CAD build for the part. Positions are in the model's coordinates, mm. A direction names the side the tool comes from. Round coordinates to 2 decimals unless told otherwise and drop trailing zeros. Loops run counter-clockwise (first coordinate to the right, second up) from the corner with the lowest first, then second, coordinate; pieces in that order, holes last.
from build123d import *

# Parameters (mm, degrees)
SKETCH1_W           = 30
SKETCH1_H           = 30
BOSS_EXTRUDE1_DEPTH = 15
SKETCH2_R           = 2.45
CUT_EXTRUDE1_DEPTH  = 46
CUT_EXTRUDE2_DEPTH  = 6.5
SKETCH4_R           = 6.4
CUT_EXTRUDE3_DEPTH  = 3.3
SKETCH5_R           = 4.95
CUT_EXTRUDE4_DEPTH  = 44.543541427
SKETCH6_R           = 1.25
FILLET1_R           = 0.5
CUT_EXTRUDE5_DEPTH  = 3.2
SKETCH9_W           = 34
SKETCH9_H           = 34
CUT_EXTRUDE7_DEPTH  = 9


with BuildPart() as part:
    # Sketch1 → Boss-Extrude1 (new body)
    with BuildSketch(Plane(origin=(0, 0, 0), x_dir=(0, 0, -1), z_dir=(1, 0, 0))):
        with Locations((15, 15)):
            Rectangle(SKETCH1_W, SKETCH1_H)
    extrude(amount=BOSS_EXTRUDE1_DEPTH)

    # Sketch2 → Cut-Extrude1 (cut, through all)
    with BuildSketch(Plane.ZY):
        with Locations((-24, 24)):
            Circle(SKETCH2_R)
        with Locations((-6, 24)):
            Circle(SKETCH2_R)
        with Locations((-6, 6)):
            Circle(SKETCH2_R)
        with Locations((-24, 6)):
            Circle(SKETCH2_R)
    extrude(amount=-CUT_EXTRUDE1_DEPTH, mode=Mode.SUBTRACT)

    # Sketch3 → Cut-Extrude2 (cut)
    with BuildSketch(Plane.ZY):
        Polygon((-7.609916554, 15), (-11.304958277, 21.4), (-18.695041723, 21.4), (-22.390083446, 15), (-18.695041723, 8.6), (-11.304958277, 8.6), align=None)
    extrude(amount=-CUT_EXTRUDE2_DEPTH, mode=Mode.SUBTRACT)

    # Sketch4 → Cut-Extrude3 (cut)
    with BuildSketch(Plane.ZY.offset(-6.5)):
        with Locations((-15, 15)):
            Circle(SKETCH4_R)
    extrude(amount=-CUT_EXTRUDE3_DEPTH, mode=Mode.SUBTRACT)

    # Sketch5 → Cut-Extrude4 (cut, through all)
    with BuildSketch(Plane.ZY.offset(-9.8)):
        with Locations((-15, 15)):
            Circle(SKETCH5_R)
    extrude(amount=-CUT_EXTRUDE4_DEPTH, mode=Mode.SUBTRACT)

    # Sketch6 → Cut-Revolve1 (revolve, cut)
    with BuildSketch(Plane.XY.offset(-15), mode=Mode.PRIVATE) as cut_revolve1_sk:
        with Locations((14.4, 23.3)):
            Circle(SKETCH6_R)
    revolve(cut_revolve1_sk.sketch.rotate(Axis((9.8, 15, -15), (-1, 0, 0)), 90), axis=Axis((9.8, 15, -15), (-1, 0, 0)), mode=Mode.SUBTRACT)

    # Fillet1
    fillet1_edges = [part.edges().sort_by_distance(p)[0] for p in [
        (0, 30, -15),
        (0, 15, -30),
        (0, 0, -15),
        (0, 15, 0),
        (7.5, 30, -30),
        (7.5, 0, -30),
    ]]
    fillet(fillet1_edges, radius=FILLET1_R)

    # Sketch7 → Cut-Extrude5 (cut)
    with BuildSketch(Plane.ZY):
        Polygon((-18.630642497, 24), (-21.315321248, 28.65), (-26.684678752, 28.65), (-29.369357503, 24), (-26.684678752, 19.35), (-21.315321248, 19.35), align=None)
        Polygon((-0.630642497, 24), (-3.315321248, 28.65), (-8.684678752, 28.65), (-11.369357503, 24), (-8.684678752, 19.35), (-3.315321248, 19.35), align=None)
        Polygon((-0.630642497, 6), (-3.315321248, 10.65), (-8.684678752, 10.65), (-11.369357503, 6), (-8.684678752, 1.35), (-3.315321248, 1.35), align=None)
        Polygon((-18.630642497, 6), (-21.315321248, 10.65), (-26.684678752, 10.65), (-29.369357503, 6), (-26.684678752, 1.35), (-21.315321248, 1.35), align=None)
    extrude(amount=-CUT_EXTRUDE5_DEPTH, mode=Mode.SUBTRACT)

    # Sketch9 → Cut-Extrude7 (cut)
    with BuildSketch(Plane(origin=(15, 0, 0), x_dir=(0, 0, -1), z_dir=(1, 0, 0))):
        with Locations((15, 15)):
            Rectangle(SKETCH9_W, SKETCH9_H)
        with BuildLine():
            ThreePointArc((10.107346068, 27.582207179), (2.146268043, 27.853731957), (2.417792821, 19.892653932))
            ThreePointArc((2.417792821, 19.892653932), (1.5, 15), (2.417792821, 10.107346068))
            ThreePointArc((2.417792821, 10.107346068), (2.146268043, 2.146268043), (10.107346068, 2.417792821))
            ThreePointArc((10.107346068, 2.417792821), (15, 1.5), (19.892653932, 2.417792821))
            ThreePointArc((19.892653932, 2.417792821), (27.853731957, 2.146268043), (27.582207179, 10.107346068))
            ThreePointArc((27.582207179, 10.107346068), (28.5, 15), (27.582207179, 19.892653932))
            ThreePointArc((27.582207179, 19.892653932), (27.853731957, 27.853731957), (19.892653932, 27.582207179))
            ThreePointArc((19.892653932, 27.582207179), (15, 28.5), (10.107346068, 27.582207179))
        make_face(mode=Mode.SUBTRACT)
    extrude(amount=-CUT_EXTRUDE7_DEPTH, mode=Mode.SUBTRACT)


solid = part.part
Item 1: Cut at C-C (z = -25.5). List the corners of the cut face in (x, y).
Verdict:
outline: (0, 0.5) arc R0.5 ccw to (0.5, 0) - (6, 0) - (6, 0.76) - (15, 0.76) - (15, 4.06) - (3.2, 4.06) - (3.2, 1.35) - (0, 1.35) - close; (0, 10.65) - (3.2, 10.65) - (3.2, 7.94) - (15, 7.94) - (15, 22.06) - (3.2, 22.06) - (3.2, 19.35) - (0, 19.35) - close; (0, 28.65) - (3.2, 28.65) - (3.2, 25.94) - (15, 25.94) - (15, 29.24) - (6, 29.24) - (6, 30) - (0.5, 30) arc R0.5 ccw to (0, 29.5) - close
Item 2: Cut at A-A (x = 5). List the corners of the cut face in (y, z), plus the area to 3 significant figures.
Verdict:
outline: (0, -29.5) arc R0.5 ccw to (0.5, -30) - (29.5, -30) arc R0.5 ccw to (30, -29.5) - (30, 0) - (0, 0) - close; hole circle Ø4.9 at (6, -24); hole circle Ø4.9 at (6, -6); hole (8.6, -18.7) - (15, -22.39) - (21.4, -18.7) - (21.4, -11.3) - (15, -7.61) - (8.6, -11.3) - close; hole circle Ø4.9 at (24, -24); hole circle Ø4.9 at (24, -6)
area: 683 mm2
Item 3: 3-axis set-ups, long thin cutter, end or side, ignore diameter. For faces 4 (the cylindrical face through (10.563, 2.059, -27.764)), 5 (the cylindrical face through (10.6, 28.5, -15.1)), 6 (the flat face through (1.578, 3.642, -1.992)), 7 (the flat face through (3, 30, -15)), 8 (the cylindrical face through (9.017, 24.108, -26.448)): which of +Z, -Z, +X, -X, +Y, -Y reach the whole face in a straight line?
Verdict:
face 4: +X
face 5: +X, +Y
face 6: -X
face 7: +Z, -Z, +X, -X, +Y
face 8: +X, -X
Item 4: Cut at B-B (y = 25). List the corners of the cut face in (x, z).
Verdict:
outline: (0, -29.5) arc R0.5 ccw to (0.5, -30) - (6, -30) - (6, -29.36) - (15, -29.36) - (15, -26.24) - (3.2, -26.24) - (3.2, -28.79) - (0, -28.79) - close; (0, -19.21) - (3.2, -19.21) - (3.2, -21.76) - (15, -21.76) - (15, -8.24) - (3.2, -8.24) - (3.2, -10.79) - (0, -10.79) - close; (0, -1.21) - (3.2, -1.21) - (3.2, -3.76) - (15, -3.76) - (15, -0.64) - (6, -0.64) - (6, 0) - (0.5, 0) arc R0.5 ccw to (0, -0.5) - close
Item 5: Mould opens along Y. For faces 1 (the flat face through (1.578, 21.708, -28.046)), 2 (the cylindrical face through (10.6, 1.5, -14.9)), 3 (the flat face through (0, 22, -15)) say: released by +Y, released by -Y, zero draft, split by the parting line, or undercut.
Verdict:
face 1: undercut
face 2: released by -Y
face 3: zero draft
Item 6: Wall check: L1, parallel to Y at x = 7.5, z = -24; L2, parallel to Y at x = 7.65, z = -15; L3, parallel to Y at x = 11.75, z = -14.75. Give the ranges that are in metal, low to high.
Verdict:
L1: y = 0.55 to 3.55, 8.45 to 21.55, 26.45 to 29.45
L2: y = 1.5 to 8.6, 21.4 to 28.5
L3: y = 1.5 to 10.06, 19.94 to 28.5
Item 7: Cut at D-D (x = 2). State how many separate pieces and enclosed holes the cut face has, plus the area to 3 significant figures.
Verdict:
separate pieces: 1
enclosed holes: 5
area: 458 mm2
Item 8: Flat gauge pins, fed straight in: P1, Ø6, axis at x = 11.5, y = 9.5, coming from the -Z side; P2, Ø2.5, axis at y = 10, z = -16.5, coming from the -X side; P3, Ø4.5, axis at y = 5.5, z = -8, coming from the -X side; P4, Ø10, axis at y = 25, z = -5, coming from the -X side. Where does each tip first touch, or does it go through?
Verdict:
P1: stops at z = -29.43
P2: stops at x = 6.5
P3: stops at x = 3.2
P4: stops at x = 0
